Geometry: see drawing. Coordinates: mm, zero at the bounding-box minimum. A direction names the side the tool comes from. Give positions to 0.01 mm unless a question says otherwise; leave off trailing zeros. Order: outer loops, then holes, each group sorted by start corner. A loop starts at its lowest first (then second) coordinate and runs counter-clockwise, first axis right, second up. Notation, with made-up numbers: (15, 81) -> (49, 81) arc R17 cw to (49, 98) -> close; hole circle Ø11 at (-16.75, 32.5). An arc over 180 degrees is marked (long way). Use one line per item in the form item = value. Start each with the question number.
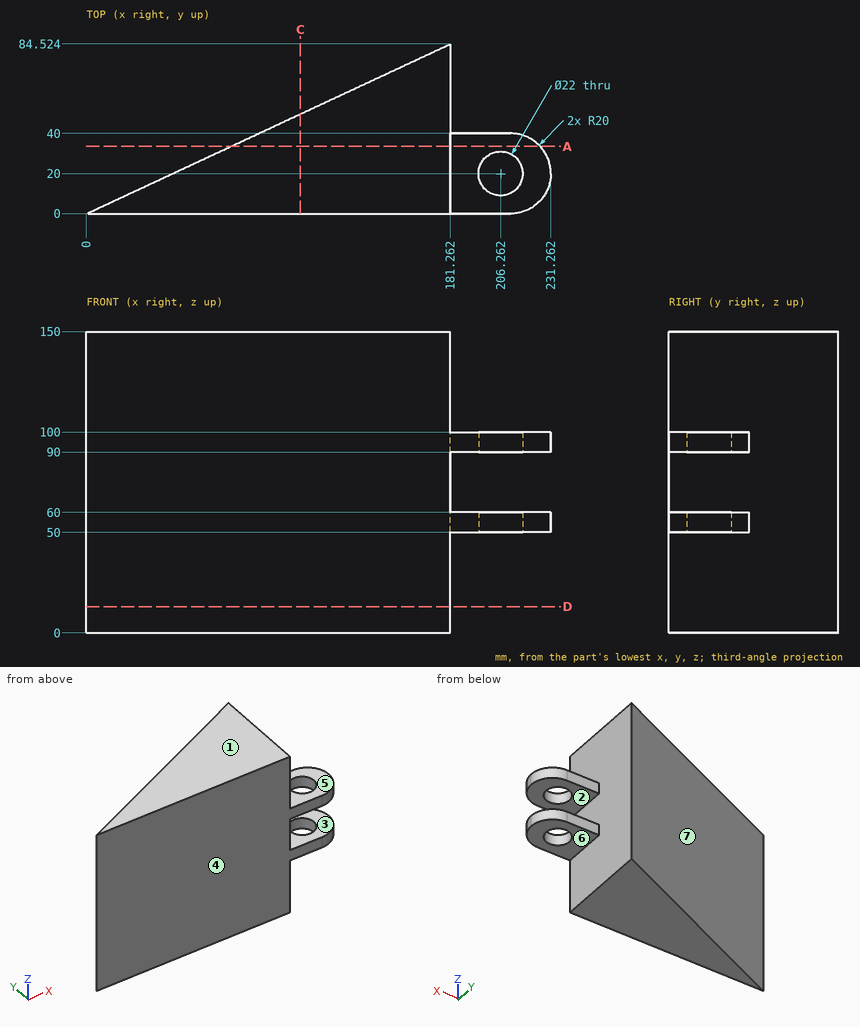
1) Pin query (flat end, axial travel): pin 1 (20 mm diameter, centred on x = 214, y = 15.5, fed in from +Z); pin 2 (5 mm diameter, centred on x = 197, z = 54.5, fed in from +Y); pin 3 (4 mm diameter, centred on x = 135.5, z = 50, fed in from +Y). Return the tip coordinate at first contact, or that it passes through.
2) Cut plane C-C, the plane x = 106.5. Return the cut outline in (y, z).
3) Reachability of the marked faces 5, 6 and 7 from +Z, -Z, +X, -X, +Y, -Y: full face, straight path, thin tool, end or side. Return the list, or none.
4) Material intervals for probe 1 along Z at (x, y) = (215, 37); probe 2 along X at (y, z) = (20, 94.75) (1 decimal); probe 3 along X at (y, z) = (24, 54) (1 decimal), sorted ascending.
5) Cut plane D-D, the plane z = 13. Return the cut outline in (x, y).
6) Draft query along Z for the marked faces 1, 2, 3 and 4. Return one class per face: +Z half, -Z half, draft (parallel to the pull), parting line (faces both ways), or undercut.
7) Cut plane A-A, the plane y = 33.5. Return the cut outline in (x, z), plus the area to 3 significant figures.
Output values:
q1.pin_1 = 100
q1.pin_2 = 40
q1.pin_3 = 64.12
q2.outline = (0, 0) -> (49.66, 0) -> (49.66, 150) -> (0, 150) -> close
q3.face_5 = +Z, +X, +Y, -Y
q3.face_6 = -Z, +X, +Y, -Y
q3.face_7 = +Z, -Z, -X, +Y
q4.probe_1 = 50 to 60, 90 to 100
q4.probe_2 = 42.9 to 195.3, 217.3 to 231.3
q4.probe_3 = 51.5 to 196, 216.5 to 230.9
q5.outline = (0, 0) -> (181.26, 0) -> (181.26, 84.52) -> close
q6.face_1 = +Z half
q6.face_2 = undercut
q6.face_3 = undercut
q6.face_4 = draft
q7.outline = (71.84, 0) -> (181.26, 0) -> (181.26, 50) -> (226.02, 50) -> (226.02, 60) -> (181.26, 60) -> (181.26, 90) -> (226.02, 90) -> (226.02, 100) -> (181.26, 100) -> (181.26, 150) -> (71.84, 150) -> close
q7.area = 17,300 mm^2
